from build123d import *

# Parameters (mm, degrees)
SKETCH_1_R          = 35.5
SKETCH_1_R_2        = 32
SKETCH_1_R_3        = 1.6
EXTRUDE_1_DEPTH     = 9
SKETCH_2_R          = 2.9
CUT_EXTRUDE_1_DEPTH = 3
CUT_EXTRUDE_3_DEPTH = 58.232752625
FILLET_START        = -1
FILLET_1_DEPTH      = 11


with BuildPart() as part:
    # 草图1 → 凸台-拉伸1 (new body)
    # profile 1 of 10: a face of its own
    with BuildSketch(Plane.XY):
        Circle(SKETCH_1_R)
        Circle(SKETCH_1_R_2, mode=Mode.SUBTRACT)
    # profile 2 of 10: a face of its own
    with BuildSketch(Plane.XY):
        with BuildLine():
            ThreePointArc((-26.073632516, 24.091817852), (-22.818960144, 27.194577731), (-19.198170234, 29.861015717))
            ThreePointArc((-19.198170234, 29.861015717), (-20.642400342, 29.576478726), (-21.890190162, 30.357364422))
            ThreePointArc((-21.890190162, 30.357364422), (-25.87220129, 30.833288836), (-26.094976213, 26.829129998))
            ThreePointArc((-26.094976213, 26.829129998), (-25.542630354, 25.46469753), (-26.073632516, 24.091817852))
        make_face()
        with Locations((-24.104535363, 28.726666617)):
            Circle(SKETCH_1_R_3, mode=Mode.SUBTRACT)
    # profile 3 of 10: a face of its own
    with BuildSketch(Plane.XY):
        with BuildLine():
            ThreePointArc((-4.48763929, 35.215211111), (0, 35.5), (4.48763929, 35.215211111))
            ThreePointArc((4.48763929, 35.215211111), (3.198397989, 35.925576349), (2.744479181, 37.325833333))
            ThreePointArc((2.744479181, 37.325833333), (0, 40.25), (-2.744479181, 37.325833333))
            ThreePointArc((-2.744479181, 37.325833333), (-3.198397989, 35.925576349), (-4.48763929, 35.215211111))
        make_face()
        with Locations((0, 37.5)):
            Circle(SKETCH_1_R_3, mode=Mode.SUBTRACT)
    # profile 4 of 10: a face of its own
    with BuildSketch(Plane.XY):
        with BuildLine():
            ThreePointArc((19.198170234, 29.861015717), (22.818960144, 27.194577731), (26.073632516, 24.091817852))
            ThreePointArc((26.073632516, 24.091817852), (25.542630354, 25.46469753), (26.094976213, 26.829129998))
            ThreePointArc((26.094976213, 26.829129998), (25.87220129, 30.833288836), (21.890190162, 30.357364422))
            ThreePointArc((21.890190162, 30.357364422), (20.642400342, 29.576478726), (19.198170234, 29.861015717))
        make_face()
        with Locations((24.104535363, 28.726666617)):
            Circle(SKETCH_1_R_3, mode=Mode.SUBTRACT)
    # profile 5 of 10: a face of its own
    with BuildSketch(Plane.XY):
        with BuildLine():
            ThreePointArc((33.900942541, 10.534519201), (34.960675232, 6.164510307), (35.459483311, 1.69559527))
            ThreePointArc((35.459483311, 1.69559527), (35.935182102, 3.088603728), (37.235343863, 3.778778563))
            ThreePointArc((37.235343863, 3.778778563), (39.638512059, 6.989339151), (36.282196246, 9.184347313))
            ThreePointArc((36.282196246, 9.184347313), (34.824390138, 9.388218001), (33.900942541, 10.534519201))
        make_face()
        with Locations((36.930290738, 6.511806663)):
            Circle(SKETCH_1_R_3, mode=Mode.SUBTRACT)
    # profile 6 of 10: a face of its own
    with BuildSketch(Plane.XY):
        with BuildLine():
            ThreePointArc((33.697359474, -16.286127976), (32.711660758, -15.192894265), (32.741087067, -13.721195927))
            ThreePointArc((32.741087067, -13.721195927), (30.743901834, -17.75), (28.253447777, -21.494015184))
            ThreePointArc((28.253447777, -21.494015184), (29.51326277, -20.732682084), (30.952880294, -21.039705357))
            ThreePointArc((30.952880294, -21.039705357), (34.857522502, -20.125), (33.697359474, -16.286127976))
        make_face()
        with Locations((32.475952642, -18.75)):
            Circle(SKETCH_1_R_3, mode=Mode.SUBTRACT)
    # profile 7 of 10: a face of its own
    with BuildSketch(Plane.XY):
        with BuildLine():
            ThreePointArc((15.3451537, -34.136142985), (15.29278176, -32.665082454), (16.261313077, -31.556610987))
            ThreePointArc((16.261313077, -31.556610987), (12.141715088, -33.359088038), (7.827310026, -34.626337054))
            ThreePointArc((7.827310026, -34.626337054), (9.281759784, -34.852915531), (10.187220033, -36.013477311))
            ThreePointArc((10.187220033, -36.013477311), (13.766310769, -37.822627987), (15.3451537, -34.136142985))
        make_face()
        with Locations((12.825755375, -35.238473279)):
            Circle(SKETCH_1_R_3, mode=Mode.SUBTRACT)
    # profile 8 of 10: a face of its own
    with BuildSketch(Plane.XY):
        with BuildLine():
            ThreePointArc((-10.187220033, -36.013477311), (-9.281759784, -34.852915531), (-7.827310026, -34.626337054))
            ThreePointArc((-7.827310026, -34.626337054), (-12.141715088, -33.359088038), (-16.261313077, -31.556610987))
            ThreePointArc((-16.261313077, -31.556610987), (-15.29278176, -32.665082454), (-15.3451537, -34.136142985))
            ThreePointArc((-15.3451537, -34.136142985), (-13.766310769, -37.822627987), (-10.187220033, -36.013477311))
        make_face()
        with Locations((-12.825755375, -35.238473279)):
            Circle(SKETCH_1_R_3, mode=Mode.SUBTRACT)
    # profile 9 of 10: a face of its own
    with BuildSketch(Plane.XY):
        with BuildLine():
            ThreePointArc((-30.952880294, -21.039705357), (-29.51326277, -20.732682084), (-28.253447777, -21.494015184))
            ThreePointArc((-28.253447777, -21.494015184), (-30.743901834, -17.75), (-32.741087067, -13.721195927))
            ThreePointArc((-32.741087067, -13.721195927), (-32.711660758, -15.192894265), (-33.697359474, -16.286127976))
            ThreePointArc((-33.697359474, -16.286127976), (-34.857522502, -20.125), (-30.952880294, -21.039705357))
        make_face()
        with Locations((-32.475952642, -18.75)):
            Circle(SKETCH_1_R_3, mode=Mode.SUBTRACT)
    # profile 10 of 10: a face of its own
    with BuildSketch(Plane.XY):
        with BuildLine():
            ThreePointArc((-35.459483311, 1.69559527), (-34.960675232, 6.164510307), (-33.900942541, 10.534519201))
            ThreePointArc((-33.900942541, 10.534519201), (-34.824390138, 9.388218001), (-36.282196246, 9.184347313))
            ThreePointArc((-36.282196246, 9.184347313), (-39.638512059, 6.989339151), (-37.235343863, 3.778778563))
            ThreePointArc((-37.235343863, 3.778778563), (-35.935182102, 3.088603728), (-35.459483311, 1.69559527))
        make_face()
        with Locations((-36.930290738, 6.511806663)):
            Circle(SKETCH_1_R_3, mode=Mode.SUBTRACT)
    extrude(amount=EXTRUDE_1_DEPTH)

    # 草图2 → 切除-拉伸1 (cut)
    with BuildSketch(Plane(origin=(0, 0, 0), x_dir=(-1, 0, 0), z_dir=(0, 0, -1))):
        with Locations((36.930290738, 6.511806663)):
            Circle(SKETCH_2_R)
        with Locations((-12.825755375, -35.238473279)):
            Circle(SKETCH_2_R)
        with Locations((-24.104535363, 28.726666617)):
            Circle(SKETCH_2_R)
    extrude(amount=-CUT_EXTRUDE_1_DEPTH, mode=Mode.SUBTRACT)

    # 草图4 → 切除-拉伸3 (cut, through all)
    with BuildSketch(Plane(origin=(0, 0, 0), x_dir=(-1, 0, 0), z_dir=(0, 0, -1))):
        with BuildLine():
            Line((15.906018141, -31.737179883), (13.847443054, -28.848714371))
            ThreePointArc((13.847443054, -28.848714371), (20.641141261, -24.45287892), (26.114981508, -18.493451297))
            Line((26.114981508, -18.493451297), (28.253447777, -21.494015184))
            ThreePointArc((28.253447777, -21.494015184), (22.665948321, -27.322239782), (15.906018141, -31.737179883))
        make_face()
    extrude(amount=-CUT_EXTRUDE_3_DEPTH, mode=Mode.SUBTRACT)

    # 圆角1: read off the stored shape, not the designer's step
    # 圆角1 outline → 圆角1 (cut)
    with BuildSketch(Plane.XY.offset(FILLET_START)):
        with BuildLine():
            ThreePointArc((-16.261313077, -31.556610987), (-15.974969952, -31.736306296), (-15.722982331, -31.961661634))
            ThreePointArc((-15.722982331, -31.961661634), (-15.818569327, -31.852738575), (-15.906018141, -31.737179883))
            ThreePointArc((-15.906018141, -31.737179883), (-16.083919009, -31.647394036), (-16.261313077, -31.556610987))
        make_face()
    extrude(amount=FILLET_1_DEPTH, mode=Mode.SUBTRACT)


solid = part.part
Input: part model. Units: mm. Frame: model coordinates. A direction names the side the tool comes from. Give positions to 0.01 mm unless a question says otherwise; leave off trailing zeros. Order: outer loops, then holes, each group sorted by start corner. A loop starts at its lowest first (then second) coordinate and runs counter-clockwise, first axis right, second up. Notation, with made-up numbers: (40, -11.75) - (99, -11.75) arc R12 ccw to (99, 1.25) - close; hole circle Ø7 at (-21.75, 15.25). An arc over 180 degrees is marked (long way). Answer as a JSON object with one key per item and string values. Group by question number.
Q1. Line query: probe 1 along Y at (x, z) = (0, 4); probe 2 along X at (y, z) = (-20, 0.75); probe 3 along Y at (x, z) = (23, 4). Output: solid intervals per line, ascending.
Q2. First-contact query: pin 1 Ø5 at (x, y) = (-36.93, 6.51) entering from -Z; pin 2 Ø1.5 at (y, z) = (-1, 7.5) entering from -X; pin 3 Ø5 at (x, z) = (-27.5, 1.5) entering from +Y. Flat tips, straight axial feed; report the tip coordinate or a pass-through.
Q3. Cut plane B-B, the plane y = 0. Output: boundary loops of the cut face in (x, z).
Q4. Mould query, pull axis Y, two halves, no side actions, for faces 1 (the face through (12.25, 33.32, 4.44)), 2 (the face through (21.1, 24.5, 0)), 3 (the face through (-34.89, -20.07, 4.44)), 4 (the face through (22.8, 27.8, 6)). Classes: pulls with the +Y half, pulls with the -Y half, needs draft (parallel to the pull), parting line crosses it, or undercut.
Q5. Set-up query: faces 5 (the face through (-34.066, 6.06, 1.479)), 6 (the face through (-12.038, 33.397, 4.437)), 7 (the face through (-38.53, 6.58, 5.96)). Return all of +Z, -Z, +X, -X, +Y, -Y with unobstructed straight access to the full face (end or side cutting, diameter ignored); none if empty.
Q6. Cut plane C-C, the plane x = -24.5. Output: boundary loops of the cut face in (y, z).
Q7. Cut plane D-D, the plane z = 6.25. Count the separate pieces of the cut face and the enclosed holes in it, then the cut area to 3 significant figures.
Q8. Cut plane A-A, the plane x = 0. Output: boundary loops of the cut face in (y, z).
Results:
{
 "1": {"probe 1": "-35.5 to -32, 32 to 35.9, 39.1 to 40.25", "probe 2": "-34.93 to -33.47, -31.48 to -27.19, 24.98 to 31.48, 33.47 to 34.93", "probe 3": "-27.04 to -22.25, 22.25 to 27.57, 29.88 to 31.25"},
 "2": {"pin 1": "z = 3", "pin 2": "x = -35.5", "pin 3": "y = 31.33"},
 "3": {"outline": "(-35.5, 0) - (-32, 0) - (-32, 9) - (-35.5, 9) - close; (32, 0) - (35.5, 0) - (35.5, 9) - (32, 9) - close"},
 "4": {"face 1": "pulls with the +Y half", "face 2": "needs draft", "face 3": "undercut", "face 4": "undercut"},
 "5": {"face 5": "-Z, -X", "face 6": "+Z, -Z, +Y", "face 7": "+Z, -Z"},
 "6": {"outline": "(20.59, 0) - (27.18, 0) - (27.18, 9) - (20.59, 9) - close; (30.28, 0) - (31.45, 0) - (31.45, 9) - (30.28, 9) - close"},
 "7": {"separate pieces": "1", "enclosed holes": "9", "area": "832 mm^2"},
 "8": {"outline": "(-35.5, 0) - (-32, 0) - (-32, 9) - (-35.5, 9) - close; (32, 0) - (35.9, 0) - (35.9, 9) - (32, 9) - close; (39.1, 0) - (40.25, 0) - (40.25, 9) - (39.1, 9) - close"}
}
